Autodesk Inventor part; units mm, degrees
ref_plane "YZ Plane" through (0, 0, 0) normal (1, 0, 0) x (0, 1, 0)
ref_plane "XZ Plane" through (0, 0, 0) normal (0, 1, 0) x (-1, 0, 0)
ref_plane "XY Plane" through (0, 0, 0) normal (0, 0, 1) x (1, 0, 0)
sketch "Sketch1" plane through (0, 0, 0) normal (1, 0, 0) x (0, 1, 0)
  point P0 (0, 0)
sketch "Sketch2" plane through (0, 0, 0) normal (1, 0, 0) x (0, 1, 0)
  line L0 (0, 0) -> (25.4, 0)
  line L1 (25.4, 0) -> (25.4, -25.4)
  line L2 (25.4, -25.4) -> (0, -25.4)
  line L3 (0, -25.4) -> (0, 0)
  dimension "d0" = 25.4
  dimension "d1" = 25.4
extrude "Extrusion1" add sketch "Sketch2" along normal blind 101.6
sketch "Sketch3" plane through (101.6, 0, 0) normal (1, 0, 0) x (0, 0, -1)
  line L0 (0, 0) -> (25.4, 0)
  line L1 (0, 0) -> (3.175, 0)
  line L2 (3.175, 0) -> (0, 0)
  line L3 (3.175, 0) -> (3.175, 3.175)
  line L4 (3.175, 3.175) -> (22.225, 3.175)
  line L5 (22.225, 3.175) -> (22.225, 22.225)
  line L6 (22.225, 22.225) -> (3.175, 22.225)
  line L7 (3.175, 22.225) -> (3.175, 3.175)
  dimension "d7" = 19.05
  dimension "d8" = 19.05
extrude "Extrusion2" cut sketch "Sketch3" against normal blind 50.8
sketch "Sketch4" plane through (0, 0, 0) normal (-1, 0, 0) x (0, 0, 1)
  line L0 (-25.4, 0) -> (-25.4, 25.4)
  line L1 (-25.4, 25.4) -> (0, 25.4)
  line L2 (-22.225, 3.175) -> (-3.175, 3.175)
  line L3 (-22.225, 22.225) -> (-22.225, 3.175)
  line L4 (-21.59, 3.302) -> (-22.098, 3.302)
  line L5 (-17.272, 8.128) -> (-8.128, 8.128)
  line L6 (-8.128, 8.128) -> (-8.128, 17.907)
  line L7 (-8.128, 17.907) -> (-17.272, 17.907)
  line L8 (-17.272, 17.907) -> (-17.272, 8.128)
  line L9 (-22.098, 3.302) -> (-3.302, 3.302)
  line L10 (-3.302, 3.302) -> (-3.302, 22.733)
  line L11 (-3.302, 22.733) -> (-22.098, 22.733)
  line L12 (-22.098, 22.733) -> (-22.098, 3.302)
extrude "Extrusion3" cut sketch "Sketch4" against normal blind 38.1
properties part number "Side Piece"
Design review of the part built by this model. Coordinates are the model's own, in mm. A direction names the side the tool comes from. Give positions to 0.01 mm unless a question says otherwise; leave off trailing zeros. Write each loop counter-clockwise with the first axis right and the second up, starting at its lowest first coordinate (ties: lowest second). Pieces come first, ordered by that corner, then holes. Notation, with made-up numbers: M 87.25,60.5 L 130.25,60.5 A8 cw 130.25,67.5 Z; hole C 29,4.5 d4. An arc over 180 degrees is marked long. Answer as a JSON object with one key per item and string values. Group by question number.
1) We need section C-C (y = 5.75). Give the boundary of the cut face in (x, z) (3 decimals).
2) We need section A-A (x = 14.5). Give the boundary of the cut face in (y, z), and give its area (3 significant figures).
3) Mouldability with a two-part tool opening along Z and no side actions: class faces 1 (the face through (50.8, 13, -13)), 2 (the face through (50, 25.4, -13)), 3 (the face through (50, 13, 0)) as released by +Z, released by -Z, zero draft, split by the parting line, or undercut.
4) We need section B-B (x = 83). Give the boundary of the cut face in (y, z) (3 decimals), and give its area (3 significant figures).
5) For line 1 along Z through (x, y) = (27, 12.75); line 2 along Y through (x, z) = (52.5, -13.25) (3 decimals); line 3 along Y through (x, z) = (19, -6.75), list the stretches that pass through material, from the lowest coordinate up.
6) We need section D-D (z = -19.25). Give the boundary of the cut face in (x, y) (3 decimals).
7) Tool access review of faces 4 (the face through (50, 0, -13)), 5 (the face through (19, 3.302, -13)), 6 (the face through (77, 13, -3.175)): name each direction out of +Z, -Z, +X, -X, +Y, -Y from which nothing blocks a thin tool from reaching the whole face with its end or side.
Answer key:
{
 "1": {"outline": "M 0,-25.4 L 101.6,-25.4 L 101.6,-22.225 L 50.8,-22.225 L 50.8,-3.175 L 101.6,-3.175 L 101.6,0 L 0,0 L 0,-3.302 L 38.1,-3.302 L 38.1,-22.098 L 0,-22.098 Z"},
 "2": {"outline": "M 0,-25.4 L 25.4,-25.4 L 25.4,0 L 0,0 Z; M 8.13,-17.27 L 17.91,-17.27 L 17.91,-8.13 L 8.13,-8.13 Z; hole M 3.3,-22.1 L 22.73,-22.1 L 22.73,-3.3 L 3.3,-3.3 Z", "area": "369 mm²"},
 "3": {"face 1": "undercut", "face 2": "zero draft", "face 3": "released by +Z"},
 "4": {"outline": "M 0,-25.4 L 25.4,-25.4 L 25.4,0 L 0,0 Z; hole M 3.175,-22.225 L 22.225,-22.225 L 22.225,-3.175 L 3.175,-3.175 Z", "area": "282 mm²"},
 "5": {"line 1": "z = -25.4 to -22.1, -17.27 to -8.13, -3.3 to 0", "line 2": "y = 0 to 3.175, 22.225 to 25.4", "line 3": "y = 0 to 3.3, 22.73 to 25.4"},
 "6": {"outline": "M 0,0 L 101.6,0 L 101.6,3.175 L 50.8,3.175 L 50.8,22.225 L 101.6,22.225 L 101.6,25.4 L 0,25.4 L 0,22.733 L 38.1,22.733 L 38.1,3.302 L 0,3.302 Z"},
 "7": {"face 4": "+Z, -Z, +X, -X, -Y", "face 5": "-X", "face 6": "+X"}
}
